```python
from build123d import *

# Parameters (mm, degrees)
SKETCH1_W               = 16.6
SKETCH1_H               = 62
BOSS_EXTRUDE1_DEPTH     = 2
SKETCH1_7_W             = 2
SKETCH1_7_H             = 41
BOSS_EXTRUDE2_DEPTH     = 12.6
SKETCH2_W               = 16.6
SKETCH2_H               = 62
BOSS_EXTRUDE3_DEPTH     = 2
SKETCH3_W               = 41
SKETCH3_H               = 8.6
CUT_EXTRUDE1_DEPTH      = 2
CUT_EXTRUDE2_DEPTH      = 2
CUT_EXTRUDE4_DEPTH      = 17.5
CUT_EXTRUDE4_DEPTH_BACK = 14.5
SKETCH5_W               = 19
SKETCH5_H               = 8.6
SKETCH5_W_2             = 2
SKETCH7_W               = 16.6
SKETCH7_H               = 4
BOSS_EXTRUDE4_DEPTH     = 2
SKETCH9_R               = 1.25
CUT_EXTRUDE6_DEPTH      = 20
FILLET3_R               = 1
CUT_EXTRUDE7_DEPTH      = 21
SKETCH13_W              = 2
SKETCH13_H              = 2
CUT_EXTRUDE8_DEPTH      = 3


with BuildPart() as part:
    # Sketch1 → Boss-Extrude1 (new body)
    with BuildSketch(Plane(origin=(0, 0, 0), x_dir=(1, 0, 0), z_dir=(0, 1, 0))):
        with Locations((8.3, 29)):
            Rectangle(SKETCH1_W, SKETCH1_H)
    extrude(amount=-BOSS_EXTRUDE1_DEPTH)

    # Sketch1_7 → Boss-Extrude2 (add)
    with BuildSketch(Plane(origin=(0, 0, 0), x_dir=(1, 0, 0), z_dir=(0, 1, 0))):
        with Locations((1, 39.5)):
            Rectangle(SKETCH1_7_W, SKETCH1_7_H)
        Polygon((0, 0), (14.6, 0), (14.6, 60), (16.6, 60), (16.6, 0), (16.6, -2), (0, -2), align=None)
    extrude(amount=BOSS_EXTRUDE2_DEPTH)

    # Sketch2 → Boss-Extrude3 (add)
    with BuildSketch(Plane(origin=(0, 12.6, 0), x_dir=(1, 0, 0), z_dir=(0, 1, 0))):
        with Locations((8.3, 29)):
            Rectangle(SKETCH2_W, SKETCH2_H)
    extrude(amount=BOSS_EXTRUDE3_DEPTH)

    # Sketch3 → Cut-Extrude1 (cut)
    with BuildSketch(Plane.ZY):
        with Locations((-39.5, 6.3)):
            Rectangle(SKETCH3_W, SKETCH3_H)
    extrude(amount=-CUT_EXTRUDE1_DEPTH, mode=Mode.SUBTRACT)

    # Sketch4 → Cut-Extrude2 (cut)
    with BuildSketch(Plane.ZY):
        with BuildLine():
            ThreePointArc((-20.999, 2), (-19.585493544, 1.414506456), (-19, 0.001))
            Line((-19, 0.001), (-19, 2))
            Line((-19, 2), (-20.999, 2))
        make_face()
        with BuildLine():
            ThreePointArc((-19, 12.599), (-19.585493544, 11.185493544), (-20.999, 10.6))
            Line((-20.999, 10.6), (-19, 10.6))
            Line((-19, 10.6), (-19, 12.599))
        make_face()
    extrude(amount=-CUT_EXTRUDE2_DEPTH, mode=Mode.SUBTRACT)

    # Sketch5 → Cut-Extrude4 (cut, two sides: drawn at the far end of the back side and taken through both)
    with BuildSketch(Plane.ZY.offset(-14.6).offset(-CUT_EXTRUDE4_DEPTH_BACK)):
        with Locations((-9.5, 6.3)):
            Rectangle(SKETCH5_W, SKETCH5_H)
        with Locations((1, 6.3)):
            Rectangle(SKETCH5_W_2, SKETCH5_H)
    extrude(amount=CUT_EXTRUDE4_DEPTH + CUT_EXTRUDE4_DEPTH_BACK, mode=Mode.SUBTRACT)

    # Sketch7 → Boss-Extrude4 (add)
    with BuildSketch(Plane.XY.offset(2)):
        with Locations((8.3, 0)):
            Rectangle(SKETCH7_W, SKETCH7_H)
        with Locations((8.3, 12.6)):
            Rectangle(SKETCH7_W, SKETCH7_H)
    extrude(amount=BOSS_EXTRUDE4_DEPTH)

    # Sketch9 → Cut-Extrude6 (cut)
    with BuildSketch(Plane(origin=(0, 14.6, 0), x_dir=(1, 0, 0), z_dir=(0, 1, 0))):
        with Locations(Location((14.6, -2, 0), (0, 0, 270))):
            Circle(SKETCH9_R)
    extrude(amount=-CUT_EXTRUDE6_DEPTH, mode=Mode.SUBTRACT)

    # Fillet3
    fillet3_edges = [part.edges().sort_by_distance(p)[0] for p in [
        (0, 1, 0),
        (0, 0, -9.5),
        (0, 11.6, 0),
        (0, 12.6, -9.5),
    ]]
    fillet(fillet3_edges, radius=FILLET3_R)

    # Sketch12 → Cut-Extrude7 (cut)
    with BuildSketch(Plane(origin=(0, -2, 0), x_dir=(-1, 0, 0), z_dir=(0, -1, 0))):
        Polygon((0, 59.999), (0, 60), (-1.99900025, 58.00000025), (-2, 57.999), (-2, 57), (0, 57), (0, 57.999), (0, 58), align=None)
    extrude(amount=-CUT_EXTRUDE7_DEPTH, mode=Mode.SUBTRACT)

    # Sketch13 → Cut-Extrude8 (cut)
    with BuildSketch(Plane(origin=(0, 0, -60), x_dir=(-1, 0, 0), z_dir=(0, 0, -1))):
        with Locations((-1, 11.6)):
            Rectangle(SKETCH13_W, SKETCH13_H)
        with Locations((-1, 1)):
            Rectangle(SKETCH13_W, SKETCH13_H)
    extrude(amount=-CUT_EXTRUDE8_DEPTH, mode=Mode.SUBTRACT)


solid = part.part
```
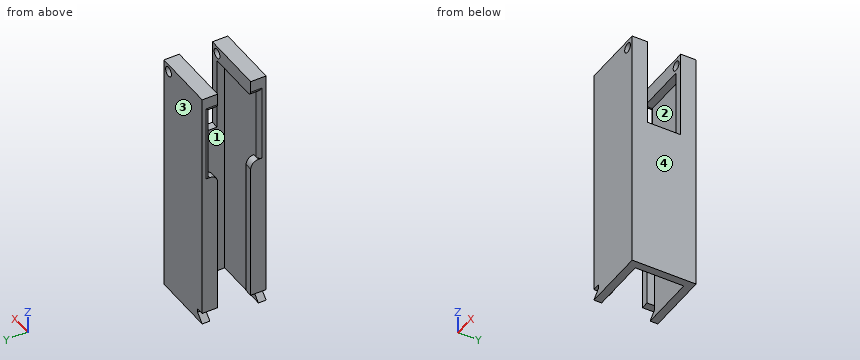
Here's how the part is built. I have some questions about the finished solid (model axes, mm). Face numbers are marked on the shaded views. Round coordinates to 2 decimals unless told otherwise and drop trailing zeros. Order: outer loops, then holes, each group sorted by start corner. A loop starts at its lowest first (then second) coordinate and runs counter-clockwise, first axis right, second up. Notation, with made-up numbers: M -28.5,4.5 L 22.5,4.5 A23 cw 22.5,28.5 Z; hole C 1,33 d2. An arc over 180 degrees is marked long. Use CSV: the item, a comma, the result in double quotes.
1) I'm going to push flat-ended pins straight in: P1, Ø0.5, axis at y = -0.5, z = -57.5, coming from the -X side; P2, Ø2, axis at y = 2, z = -50.5, coming from the -X side; P3, Ø2, axis at x = 14.6, z = 2, coming from the +Y side; P4, Ø2, axis at x = 15.5, y = 5, coming from the +Z side. Where does each tip first touch, or does it pass through?
Taken from the geometry:
P1,"x = 2"
P2,"x = 0"
P3,"through"
P4,"z = -19"
2) I need wall thicknesses on line 1 along Y through (x, z) = (9.5, -0.5); line 2 along X through (y, z) = (12.7, 2); line 3 along Y through (x, z) = (15, -16). Which ranges of each line are inside material? Lowest first, please. Write a range as [from, to].
Taken from the geometry:
line 1,"[-2, 0], [12.6, 14.6]"
line 2,"[0, 13.35], [15.85, 16.6]"
line 3,"[-2, 2], [10.6, 14.6]"
3) I want a section at A-A (z = 2). List the corners of the cut face in (x, y) for me.
Taken from the geometry:
outline,"M 0,-2 L 13.35,-2 L 13.35,2 L 0,2 Z; M 0,10.6 L 13.35,10.6 L 13.35,14.6 L 0,14.6 Z; M 15.85,-2 L 16.6,-2 L 16.6,2 L 15.85,2 Z; M 15.85,10.6 L 16.6,10.6 L 16.6,14.6 L 15.85,14.6 Z"
4) I want a section at D-D (z = -5). List the corners of the cut face in (x, y) for me, then the cut area to 3 significant figures.
Taken from the geometry:
outline,"M 0,-2 L 16.6,-2 L 16.6,2 L 14.6,2 L 14.6,0 L 1,0 A1 ccw 0,-1 Z; M 0,13.6 A1 ccw 1,12.6 L 14.6,12.6 L 14.6,10.6 L 16.6,10.6 L 16.6,14.6 L 0,14.6 Z"
area,"74.0 mm^2"
5) I want a section at B-B (y = 1). List the corners of the cut face in (x, z) for me.
Taken from the geometry:
outline,"M 0,-57 L 2,-57 L 2,-19.27 L 0,-19.27 Z; M 0,1 A1 ccw 1,0 L 14.6,0 L 14.6,-60 L 16.6,-60 L 16.6,4 L 0,4 Z; hole C 14.6,2 d2.5"
6) I want a section at C-C (x = 4.75). List the corners of the cut face in (y, z) for me.
Taken from the geometry:
outline,"M -2,-60 L 0,-60 L 0,0 L 2,0 L 2,4 L -2,4 Z; M 10.6,0 L 12.6,0 L 12.6,-60 L 14.6,-60 L 14.6,4 L 10.6,4 Z"
7) If we mould it in two halves opening along Y, with no side actions, what happens to the marked faces 1, 2, 3 and 4? For each: pulls with the +Y half, pulls with the -Y half, needs draft (parallel to the pull), parting line crosses it, or undercut.
Taken from the geometry:
face 1,"undercut"
face 2,"undercut"
face 3,"pulls with the +Y half"
face 4,"needs draft"
